Here's how the part is built. I have some questions about the finished solid (model axes, mm). Give positions to 0.01 mm unless a question says otherwise; leave off trailing zeros. Order: outer loops, then holes, each group sorted by start corner. A loop starts at its lowest first (then second) coordinate and runs counter-clockwise, first axis right, second up. Notation, with made-up numbers: M 12,50 L 33,50 A34 cw 33,85 Z; hole C 63.25,-30 d3. An arc over 180 degrees is marked long. Use CSV: the item, a comma, the result in double quotes. Start each with the question number.
```python
from build123d import *

# Parameters (mm, degrees)
BOSS_EXTRUDE1_DEPTH = 10
SKETCH2_R           = 16.25
BOSS_EXTRUDE2_DEPTH = 10
SKETCH3_R           = 16.25
CUT_EXTRUDE4_DEPTH  = 10


with BuildPart() as part:
    # Sketch1 → Boss-Extrude1 (new body)
    with BuildSketch(Plane.XY):
        with BuildLine():
            ThreePointArc((-150, 25), (-175, 0), (-150, -25))
            ThreePointArc((-150, -25), (0, -13.685996664), (150, -25))
            ThreePointArc((150, -25), (175, 0), (150, 25))
            ThreePointArc((150, 25), (0, 13.685996664), (-150, 25))
        make_face()
    extrude(amount=BOSS_EXTRUDE1_DEPTH)

    # Sketch2 → Boss-Extrude2 (add)
    with BuildSketch(Plane(origin=(0, 0, 0), x_dir=(1, 0, 0), z_dir=(0, 0, -1))):
        with Locations((-150, 0)):
            Circle(SKETCH2_R)
    extrude(amount=BOSS_EXTRUDE2_DEPTH)

    # Sketch3 → Cut-Extrude4 (cut)
    with BuildSketch(Plane.XY.offset(10)):
        with Locations((150, 0)):
            Circle(SKETCH3_R)
    extrude(amount=-CUT_EXTRUDE4_DEPTH, mode=Mode.SUBTRACT)


solid = part.part
```
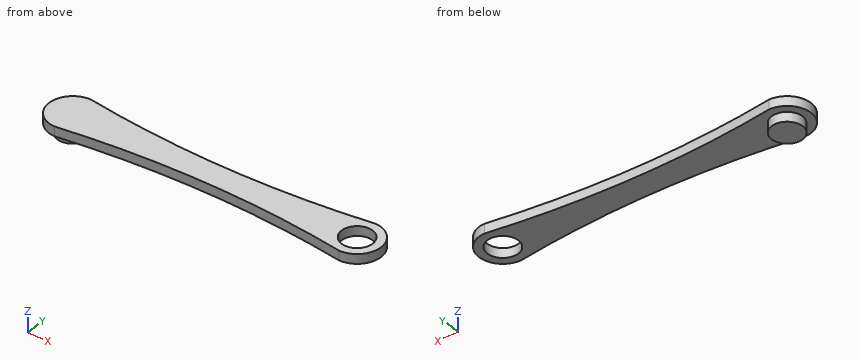
Q1. For P1, Ø6, axis at x = 52, y = -5, coming from the -Z side; P2, Ø2, axis at y = 18, z = 4.5, coming from the -X side; P3, Ø1.5, axis at x = -52, y = -16, coming from the +Z side; P4, Ø3, axis at x = 93, z = 4.5, coming from the -Y side, each with a flat end and sliding along its axis, tell me the tip position at first contact or that it passes through.
Q2. Imagine slicing it at A-A, the plane y = 0. Please give me the cut outline in (x, z).
Q3. Imagine slicing it at D-D, the plane x = -116.5. Please give me the cut outline in (y, z).
Q4. Imagine slicing it at B-B, the plane z = -3.5. Please give me the cut outline in (x, y).
Q5. I need wall thicknesses on line 1 (Y direction, x = 150, z = 4); line 2 (Z direction, x = 91, y = 8.5); line 3 (X direction, y = -5, z = 6.5). Which ranges of each line are inside material? Lowest first, please. Write a range as [from, to].
Q6. Imagine slicing it at C-C, the plane y = 21. Please give me the cut outline in (x, z).
Reply:
1,P1,"stops at z = 0"
1,P2,"stops at x = -168.33"
1,P3,"passes through"
1,P4,"stops at y = -18.16"
2,outline,"M -175,0 L -166.25,0 L -166.25,-10 L -133.75,-10 L -133.75,0 L 133.75,0 L 133.75,10 L -175,10 Z; M 166.25,0 L 175,0 L 175,10 L 166.25,10 Z"
3,outline,"M -20.5,0 L 20.5,0 L 20.5,10 L -20.5,10 Z"
4,outline,"C -150,0 d32.5"
5,line 1,"y = [-25, -16.25], [16.25, 25]"
5,line 2,"z = [0, 10]"
5,line 3,"x = [-174.49, 134.54], [165.46, 174.49]"
6,outline,"M -163.56,0 L -120.72,0 L -120.72,10 L -163.56,10 Z; M 120.72,0 L 163.56,0 L 163.56,10 L 120.72,10 Z"
